The model under review builds one solid part; all positions refer to its coordinate system, in mm. Face numbers are marked on the shaded views. Coordinates: 2 decimals unless noted, no trailing zeros. Order: outer loops, then holes, each group sorted by start corner. A loop starts at its lowest first (then second) coordinate and runs counter-clockwise, first axis right, second up. Notation, with made-up numbers: M -27.75,82.5 L 8.25,82.5 A31 cw 8.25,114.5 Z; hole C 40,33.5 d11. An arc over 180 degrees is marked long. Answer as CSV lines item,"result". Start each with the question number.
Q1. Consider section A-A on x = -20. Write out the cut boundary in (y, z).
Q2. For P1, Ø5, axis at x = -0.5, y = 6, coming from the +Z side; P2, Ø4, axis at y = 1.5, z = -35.5, coming from the +X side; P3, Ø4, axis at y = 5, z = -63, coming from the -X side; P4, Ø6, axis at x = 2, y = 4.5, coming from the -Z side, all flat-tipped, find the tip position at first contact; note any pin that passes through.
Q3. Consider section C-C on y = 9. Write out the cut boundary in (x, z), and give its area (3 significant figures).
Q4. Consider section D-D on x = 12. Write out the cut boundary in (y, z).
Q5. Consider section B-B on z = -10. Write out the cut boundary in (x, y).
Q6. Wall thickness on L1, parallel to X at y = 3.5, z = -14.5; L2, parallel to X at y = 7, z = -61.5; L3, parallel to Y at x = -9.25, z = -63: over which ranges is each line inside the solid? List them lowest first. Write a range as [from, to].
Q7. The part is to be moulded in two halves that separate along X. For the marked faces 1, 2 and 3, say which applies: +X half, -X half, draft (parallel to the pull), parting line (faces both ways), or undercut.
from build123d import *

# Parameters (mm, degrees)
SKETCH_1_W               = 50
SKETCH_1_H               = 43
EXTRUDE_1_DEPTH          = 5
SKETCH_3_R               = 5
EXTRUDE_2_DEPTH          = 5
EXTRUDE_START            = -6
EXTRUDE_3_DEPTH          = 5
EXTRUDE_4_DEPTH          = 5
SKETCH_9_R               = 1.5
CUT_EXTRUDE_2_DEPTH      = 11
CUT_EXTRUDE_2_DEPTH_BACK = 41
SKETCH_11_W              = 3
SKETCH_11_H              = 11
SKETCH_11_W_2            = 6
SKETCH_11_W_3            = 16
SKETCH_11_W_4            = 10
CUT_EXTRUDE_3_DEPTH      = 6
CUT_EXTRUDE_3_DEPTH_BACK = 6
SKETCH_12_R              = 1.5
CUT_EXTRUDE_4_DEPTH      = 32
CUT_EXTRUDE_4_DEPTH_BACK = 20
SKETCH_13_W              = 10
SKETCH_13_H              = 32
CUT_EXTRUDE_5_DEPTH      = 6
CUT_EXTRUDE_5_DEPTH_BACK = 6
CHAMFER_2_SIZE           = 2


with BuildPart() as part:
    # 草图1 → 凸台-拉伸1 (new body)
    with BuildSketch(Plane(origin=(0, 0, 0), x_dir=(1, 0, 0), z_dir=(0, 1, 0))):
        with Locations((0, -3.5)):
            Rectangle(SKETCH_1_W, SKETCH_1_H)
    extrude(amount=EXTRUDE_1_DEPTH)

    # 草图3 → 凸台-拉伸2 (add)
    with BuildSketch(Plane(origin=(15, 0, 0), x_dir=(0, 0, -1), z_dir=(1, 0, 0))):
        with Locations((18, 5)):
            Circle(SKETCH_3_R)
    extrude(amount=-EXTRUDE_2_DEPTH)

    # 草图5 → 凸台-拉伸3 (add)
    with BuildSketch(Plane(origin=(0, 0, 0), x_dir=(0, 0, -1), z_dir=(1, 0, 0)).offset(EXTRUDE_START)):
        with BuildLine():
            Line((18, 10), (63, 10))
            ThreePointArc((63, 10), (68, 5), (63, 0))
            Line((63, 0), (18, 0))
            ThreePointArc((18, 0), (13, 5), (18, 10))
        make_face()
    extrude(amount=-EXTRUDE_3_DEPTH)

    # 草图6 → 凸台-拉伸4 (add)
    with BuildSketch(Plane(origin=(-22, 0, 0), x_dir=(0, 0, -1), z_dir=(1, 0, 0))):
        with BuildLine():
            Line((18, 10), (63, 10))
            ThreePointArc((63, 10), (68, 5), (63, 0))
            Line((63, 0), (18, 0))
            ThreePointArc((18, 0), (13, 5), (18, 10))
        make_face()
    extrude(amount=EXTRUDE_4_DEPTH)

    # 草图9 → 切除-拉伸2 (cut, two sides)
    with BuildSketch(Plane(origin=(15, 0, 0), x_dir=(0, 0, -1), z_dir=(1, 0, 0))) as cut_extrude_2_sk:
        with Locations((18, 5)):
            Circle(SKETCH_9_R)
    extrude(amount=CUT_EXTRUDE_2_DEPTH, mode=Mode.SUBTRACT)
    extrude(cut_extrude_2_sk.sketch, amount=-CUT_EXTRUDE_2_DEPTH_BACK, mode=Mode.SUBTRACT)

    # 草图11 → 切除-拉伸3 (cut, two sides)
    with BuildSketch(Plane(origin=(0, 5, 0), x_dir=(1, 0, 0), z_dir=(0, 1, 0))) as cut_extrude_3_sk:
        with Locations((-23.5, 12.5)):
            Rectangle(SKETCH_11_W, SKETCH_11_H)
        with Locations((-14, 12.5)):
            Rectangle(SKETCH_11_W_2, SKETCH_11_H)
        with Locations((2, 12.5)):
            Rectangle(SKETCH_11_W_3, SKETCH_11_H)
        with Locations((20, 12.5)):
            Rectangle(SKETCH_11_W_4, SKETCH_11_H)
    extrude(amount=CUT_EXTRUDE_3_DEPTH, mode=Mode.SUBTRACT)
    extrude(cut_extrude_3_sk.sketch, amount=-CUT_EXTRUDE_3_DEPTH_BACK, mode=Mode.SUBTRACT)

    # 草图12 → 切除-拉伸4 (cut, two sides)
    with BuildSketch(Plane(origin=(-6, 0, 0), x_dir=(0, 0, -1), z_dir=(1, 0, 0))) as cut_extrude_4_sk:
        with Locations((63, 5)):
            Circle(SKETCH_12_R)
    extrude(amount=CUT_EXTRUDE_4_DEPTH, mode=Mode.SUBTRACT)
    extrude(cut_extrude_4_sk.sketch, amount=-CUT_EXTRUDE_4_DEPTH_BACK, mode=Mode.SUBTRACT)

    # 草图13 → 切除-拉伸5 (cut, two sides)
    with BuildSketch(Plane(origin=(0, 5, 0), x_dir=(1, 0, 0), z_dir=(0, 1, 0))) as cut_extrude_5_sk:
        with Locations((20, -9)):
            Rectangle(SKETCH_13_W, SKETCH_13_H)
    extrude(amount=CUT_EXTRUDE_5_DEPTH, mode=Mode.SUBTRACT)
    extrude(cut_extrude_5_sk.sketch, amount=-CUT_EXTRUDE_5_DEPTH_BACK, mode=Mode.SUBTRACT)

    # 倒角2
    chamfer_2_edges = [part.edges().sort_by_distance(p)[0] for p in [
        (-25, 2.5, -7),
        (15, 2.5, 25),
        (-25, 2.5, 25),
    ]]
    chamfer(chamfer_2_edges, length=CHAMFER_2_SIZE)


solid = part.part
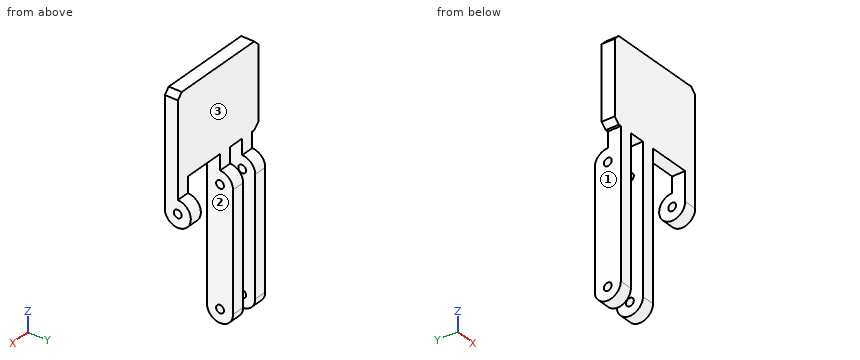
Evaluation:
1,outline,"M 0,-63 A5 ccw 10,-63 L 10,-18 A5 ccw 5,-13 L 5,25 L 0,25 Z; hole C 5,-63 d3; hole C 5,-18 d3"
2,P1,"stops at z = 25"
2,P2,"stops at x = -6"
2,P3,"stops at x = -22"
2,P4,"stops at z = -7"
3,outline,"M -22,-66 L -17,-66 L -17,-15 L -22,-15 Z; M -11,-66 L -6,-66 L -6,-15 L -11,-15 Z; M 10,-21 L 15,-21 L 15,-15 L 10,-15 Z"
3,area,"540 mm²"
4,outline,"M 0,-18 A5 ccw long 5,-13 L 5,25 L 0,25 Z; hole C 5,-18 d3"
5,outline,"M -22,0 L -17,0 L -17,5 L -22,5 Z; M -11,0 L -6,0 L -6,5 L -11,5 Z; M 10,0 L 15,0 L 15,5 L 10,5 Z"
6,L1,"x = [-22, -17], [-11, -6], [10, 15]"
6,L2,"x = [-22, -17], [-11, -6]"
6,L3,"y = [0, 3.5], [6.5, 10]"
7,face 1,"-X half"
7,face 2,"undercut"
7,face 3,"draft"
